CAD build for the part. Positions are in the model's coordinates, mm. A direction names the side the tool comes from. Coordinates: 2 decimals unless noted, no trailing zeros. Order: outer loops, then holes, each group sorted by start corner. A loop starts at its lowest first (then second) coordinate and runs counter-clockwise, first axis right, second up. Notation, with made-up numbers: (68.5, 3) - (100.5, 3) arc R12 cw to (100.5, 10) - close; hole circle Ø11 at (18, -15). An arc over 180 degrees is marked (long way). Return JSON: item names as keys, results as strings.
Autodesk Inventor part; units mm, degrees
ref_plane "YZ Plane" through (0, 0, 0) normal (1, 0, 0) x (0, 1, 0)
ref_plane "XZ Plane" through (0, 0, 0) normal (0, 1, 0) x (-1, 0, 0)
ref_plane "XY Plane" through (0, 0, 0) normal (0, 0, 1) x (1, 0, 0)
sketch "Sketch1" plane through (0, 0, 0) normal (0, 1, 0) x (-1, 0, 0)
  line L0 (-2, -229.675) -> (-6, -229.675)
  line L1 (-6, -200.675) -> (-2, -200.675)
  line L2 (0, -202.675) -> (0, -227.675)
  line L3 (-6, -30.675) -> (-2, -30.675)
  line L4 (0, -28.675) -> (0, -3.675)
  line L5 (-2, -1.675) -> (-6, -1.675)
  arc A0 (0, -3.675) -> (-2, -1.675) centre (-2, -3.675) ccw
  arc A1 (-2, -30.675) -> (0, -28.675) centre (-2, -28.675) ccw
  arc A2 (0, -202.675) -> (-2, -200.675) centre (-2, -202.675) ccw
  arc A3 (-2, -229.675) -> (0, -227.675) centre (-2, -227.675) ccw
  line L6 (-136.5, -229.675) -> (-132.5, -229.675)
  line L7 (-132.5, -200.675) -> (-136.5, -200.675)
  line L8 (-138.5, -202.675) -> (-138.5, -227.675)
  line L9 (-136.5, -30.675) -> (-132.5, -30.675)
  line L10 (-132.5, -1.675) -> (-136.5, -1.675)
  line L11 (-138.5, -3.675) -> (-138.5, -28.675)
  arc A4 (-136.5, -1.675) -> (-138.5, -3.675) centre (-136.5, -3.675) ccw
  arc A5 (-138.5, -28.675) -> (-136.5, -30.675) centre (-136.5, -28.675) ccw
  arc A6 (-136.5, -200.675) -> (-138.5, -202.675) centre (-136.5, -202.675) ccw
  arc A7 (-138.5, -227.675) -> (-136.5, -229.675) centre (-136.5, -227.675) ccw
  line L12 (-27.75, -250) -> (-27.75, -247)
  line L13 (-110.75, -250) -> (-110.75, -247)
  line L14 (-30.75, -253) -> (-107.75, -253)
  line L15 (0, -215.175) -> (-138.5, -215.175) construction
  line L16 (-113.75, -244) -> (-120.45, -244)
  line L17 (-123.45, -247) -> (-123.45, -250)
  line L18 (-126.45, -253) -> (-127.7679, -253)
  line L19 (-24.75, -244) -> (-18.05, -244)
  line L20 (-15.05, -247) -> (-15.05, -250)
  line L21 (-12.05, -253) -> (-8, -253)
  arc A8 (-15.05, -250) -> (-12.05, -253) centre (-12.05, -250) ccw
  arc A9 (-15.05, -247) -> (-18.05, -244) centre (-18.05, -247) ccw
  arc A10 (-24.75, -244) -> (-27.75, -247) centre (-24.75, -247) ccw
  arc A11 (-30.75, -253) -> (-27.75, -250) centre (-30.75, -250) ccw
  arc A12 (-110.75, -250) -> (-107.75, -253) centre (-107.75, -250) ccw
  arc A13 (-110.75, -247) -> (-113.75, -244) centre (-113.75, -247) ccw
  arc A14 (-120.45, -244) -> (-123.45, -247) centre (-120.45, -247) ccw
  arc A15 (-126.45, -253) -> (-123.45, -250) centre (-126.45, -250) ccw
  line L22 (-7.5, 0) -> (-128.9984, 0)
  line L23 (-6, -229.675) -> (-6, -251)
  line L24 (-6, -30.675) -> (-6, -200.675)
  line L25 (-132.5, -30.675) -> (-132.5, -200.675)
  line L26 (-132.5, -229.675) -> (-132.5, -91)
  line L27 (-128.9984, 0) -> (-131.5, 0)
  line L28 (-132.5, -1) -> (-132.5, -1.675)
  arc A16 (-131.5, 0) -> (-132.5, -1) centre (-131.5, -1) ccw
  line L29 (-6, -1.675) -> (-6, -1)
  line L30 (-6, 0) -> (-6, 0)
  line L31 (-7, 0) -> (-7.5, 0)
  arc A17 (-6, -1) -> (-7, 0) centre (-7, -1) ccw
  line L32 (-132.5, -91) -> (-132.5, -251)
  line L33 (-130.5, -253) -> (-127.109, -253)
  arc A18 (-132.5, -251) -> (-130.5, -253) centre (-130.5, -251) ccw
  line L34 (-4.5, -253) -> (-10.025, -253)
  arc A19 (-8, -253) -> (-6, -251) centre (-8, -251) ccw
  point P0 (0, 0)
  point P1 (0, -229.675)
  point P2 (-4, -229.675)
  point P3 (-138.5, -200.675)
  point P4 (-138.5, -30.675)
  point P5 (-134.5, -229.675)
  point P6 (-132.5, -253)
  point P7 (-27.75, -253)
  point P8 (-27.75, -244)
  point P9 (-110.75, -253)
  point P10 (-110.75, -244)
  point P11 (-69.25, -253)
  point P12 (-69.25, -215.175)
  point P13 (-123.45, -244)
  point P14 (-15.05, -244)
  point P15 (-6.4873, -253)
  point P16 (-6, -91.775)
  point P17 (-4, -1.675)
  point P18 (-134.5, -1.675)
  point P19 (0, -16.175)
  point P20 (-6, -240.3375)
  point P21 (-6, -115.675)
  point P22 (-132.5, -160.3375)
  point P23 (-132.5, -115.675)
  point P24 (-138.5, -16.175)
  point P25 (-132.5, -1.3375)
  point P26 (-134.5, -30.675)
  point P27 (-4, -30.675)
  point P28 (-4, -200.675)
  point P29 (-134.5, -200.675)
  dimension "d3" = 6
  dimension "d8" = 2
  dimension "d11" = 2
  dimension "d12" = 2
  dimension "d13" = 9
  dimension "d14" = 83
  dimension "d15" = 12.7
  dimension "d16" = 12.7
  dimension "d18" = 3
  dimension "d19" = 3
  dimension "d24" = 6
  dimension "d25" = 1
  dimension "d26" = 1
  dimension "d29" = 29
  dimension "d30" = 23.325
  dimension "d31" = 2
  dimension "d34" = 2
  dimension "d35" = 126.5
  dimension "d36" = 244
  dimension "d37" = 29
  dimension "d38" = 1.675
extrude "Extrusion1" add sketch "Sketch1" along normal blind 5
equation "\"d19\" = d18"
equation "\"d24\" = d3"
equation "\"d25\" = d26"
equation "\"d31\" = d17"
properties part number "back_wall"
Item 1: Wall check: L1, parallel to X at y = 2.85, z = -163.5; L2, parallel to Z at x = 115, y = 3.7; L3, parallel to Z at x = 26.5, y = 2.75. Give the ranges that are in metal, low to high. Write a range as [from, to].
Findings below:
{"L1": "x = [6, 132.5]", "L2": "z = [-244, 0]", "L3": "z = [-244.56, 0]"}
Item 2: Mould opens along X. For faces 5 (the flat face through (6, 2, -114)), 6 (the flat face through (21, 2, -244)), 7 (the flat face through (68, 2, 0)) say: released by +X, released by -X, zero draft, split by the parting line, or undercut.
Findings below:
{"face 5": "released by -X", "face 6": "undercut", "face 7": "zero draft"}
Item 3: Band-saw the part on A-A, the plane z = -169.5. List the corners of the cut face in (x, y).
Findings below:
{"outline": "(6, 0) - (132.5, 0) - (132.5, 5) - (6, 5) - close"}
Item 4: Which spindle directions (+Z, -Z, +X, -X, +Y, -Y) get a long thin tool onto all of the face, cutting with end or side? Do faces 1 (the flat face through (132.5, 2, -240)), 2 (the flat face through (117, 2, -244)), 3 (the flat face through (6, 2, -240)), 4 (the flat face through (132.5, 2, -114)). Say none if no direction does.
Findings below:
{"face 1": "-Z, +X, +Y, -Y", "face 2": "-Z, +Y, -Y", "face 3": "-Z, -X, +Y, -Y", "face 4": "+X, +Y, -Y"}
Item 5: Drop flat-ended pins along their axis: P1, Ø1.2, axis at x = 135, y = 2, coming from the -Z side (3 decimals); P2, Ø2.5, axis at y = 3.5, z = -249, coming from the -X side; P3, Ø1.2, axis at x = 4, y = 1.5, coming from the +Z side (3 decimals). Give the stop position or say it passes through.
Findings below:
{"P1": "stops at z = -229.675", "P2": "stops at x = 6", "P3": "stops at z = -1.675"}
